```python
from build123d import *

# Parameters (mm, degrees)
SKETCH1_W           = 80
SKETCH1_H           = 76.35
SKETCH1_R           = 32.5
SKETCH1_R_2         = 2.15
BOSS_EXTRUDE1_DEPTH = 3.175


with BuildPart() as part:
    # Sketch1 → Boss-Extrude1 (new body)
    with BuildSketch(Plane.XY):
        Rectangle(SKETCH1_W, SKETCH1_H)
        Circle(SKETCH1_R, mode=Mode.SUBTRACT)
        with Locations((-32, 24.2)):
            Circle(SKETCH1_R_2, mode=Mode.SUBTRACT)
        with Locations(Location((-32, -24.2, 0), (0, 0, 180))):
            Circle(SKETCH1_R_2, mode=Mode.SUBTRACT)
        with Locations((32, -24.2)):
            Circle(SKETCH1_R_2, mode=Mode.SUBTRACT)
        with Locations(Location((32, 24.2, 0), (0, 0, 180))):
            Circle(SKETCH1_R_2, mode=Mode.SUBTRACT)
    extrude(amount=BOSS_EXTRUDE1_DEPTH)


solid = part.part
```
Work out the finished part from the listing and answer in its coordinate system (mm). Coordinates: 2 decimals unless noted, no trailing zeros. Loops run counter-clockwise (first coordinate to the right, second up) from the corner with the lowest first, then second, coordinate; pieces in that order, holes last. Notation, with made-up numbers: M 56.5,89.5 L 63.5,89.5 A20 cw 63.5,102.5 Z; hole C -1,40.25 d1. An arc over 180 degrees is marked long. Use CSV: the item, a comma, the result in double quotes. Start each with the question number.
(1) Find section A-A, the plane y = 0. Give the vertices of the cut face in (x, z) (3 decimals), then the cut area to 3 significant figures.
(2) Find section D-D, the plane y = -24.2. Give the vertices of the cut face in (x, z) (3 decimals).
(3) Find section C-C, the plane z = 1.1. Give the vertices of the cut face in (x, y) (3 decimals).
(4) For a pull along X with two mould halves and no side action, classify faces 1 (the face through (-1, -33, 3.175)), 2 (the face through (-40, -1, 2)), 3 (the face through (-31.01, 22.29, 1.57)) as +X half, -X half, draft (parallel to the pull), parting line (faces both ways), or undercut.
(5) Find section B-B, the plane x = 0. Give the vertices of the cut face in (y, z) (3 decimals), then the cut area to 3 significant figures.
(6) Consider line 1 (Y direction, x = 19, z = 0.75) (3 decimals); line 2 (Y direction, x = 0, z = 1.1) (3 decimals); line 3 (X direction, y = 2.5, z = 2.2). Determine where each line is inside the solid, lowest interval first.
Recorded:
1,outline,"M -40,0 L -32.5,0 L -32.5,3.175 L -40,3.175 Z; M 32.5,0 L 40,0 L 40,3.175 L 32.5,3.175 Z"
1,area,"47.6 mm^2"
2,outline,"M -40,0 L -34.15,0 L -34.15,3.175 L -40,3.175 Z; M -29.85,0 L -21.694,0 L -21.694,3.175 L -29.85,3.175 Z; M 21.694,0 L 29.85,0 L 29.85,3.175 L 21.694,3.175 Z; M 34.15,0 L 40,0 L 40,3.175 L 34.15,3.175 Z"
3,outline,"M -40,-38.175 L 40,-38.175 L 40,38.175 L -40,38.175 Z; hole C -32,-24.2 d4.3; hole C -32,24.2 d4.3; hole C 0,0 d65; hole C 32,-24.2 d4.3; hole C 32,24.2 d4.3"
4,face 1,"draft"
4,face 2,"-X half"
4,face 3,"undercut"
5,outline,"M -38.175,0 L -32.5,0 L -32.5,3.175 L -38.175,3.175 Z; M 32.5,0 L 38.175,0 L 38.175,3.175 L 32.5,3.175 Z"
5,area,"36.0 mm^2"
6,line 1,"y = -38.175 to -26.368, 26.368 to 38.175"
6,line 2,"y = -38.175 to -32.5, 32.5 to 38.175"
6,line 3,"x = -40 to -32.4, 32.4 to 40"
